from build123d import *

# Parameters (mm, degrees)
BOSS_EXTRUDE1_START = -242.545742
SKETCH1_R           = 25
BOSS_EXTRUDE1_DEPTH = 21.000001
BOSS_EXTRUDE2_START = -1.7
SKETCH4_R           = 25
SKETCH4_R_2         = 17
BOSS_EXTRUDE2_DEPTH = 1.7
FILLET1_R           = 4


with BuildPart() as part:
    # Sketch1 → Boss-Extrude1 (new body)
    with BuildSketch(Plane.XY.offset(BOSS_EXTRUDE1_START)):
        with Locations(Location((0, 0, 0), (0, 0, 270))):
            Circle(SKETCH1_R)
        with BuildLine():
            Line((-21.875959298, -8.922578372), (-20.951151281, -10.918757254))
            Line((-20.951151281, -10.918757254), (-20.019493054, -10.487130107))
            ThreePointArc((-20.019493054, -10.487130107), (-13.008740953, -18.480602231), (-3.118771073, -22.383772403))
            Line((-3.118771073, -22.383772403), (-3.210800112, -23.40642567))
            Line((-3.210800112, -23.40642567), (-1.019654481, -23.603607875))
            Line((-1.019654481, -23.603607875), (-0.927625442, -22.580954609))
            ThreePointArc((-0.927625442, -22.580954609), (9.500300533, -20.506201252), (17.825529997, -13.892821179))
            Line((17.825529997, -13.892821179), (18.665159186, -14.483847298))
            Line((18.665159186, -14.483847298), (19.931496801, -12.684850621))
            Line((19.931496801, -12.684850621), (19.091867612, -12.093824502))
            ThreePointArc((19.091867612, -12.093824502), (22.509041486, -2.025599021), (20.94430107, 8.490951224))
            Line((20.94430107, 8.490951224), (21.875959298, 8.922578372))
            Line((21.875959298, 8.922578372), (20.951151281, 10.918757254))
            Line((20.951151281, 10.918757254), (20.019493054, 10.487130107))
            ThreePointArc((20.019493054, 10.487130107), (13.008740953, 18.480602231), (3.118771073, 22.383772403))
            Line((3.118771073, 22.383772403), (3.210800112, 23.40642567))
            Line((3.210800112, 23.40642567), (1.019654481, 23.603607875))
            Line((1.019654481, 23.603607875), (0.927625442, 22.580954609))
            ThreePointArc((0.927625442, 22.580954609), (-9.500300533, 20.506201252), (-17.825529997, 13.892821179))
            Line((-17.825529997, 13.892821179), (-18.665159186, 14.483847298))
            Line((-18.665159186, 14.483847298), (-19.931496801, 12.684850621))
            Line((-19.931496801, 12.684850621), (-19.091867612, 12.093824502))
            ThreePointArc((-19.091867612, 12.093824502), (-22.509041486, 2.025599021), (-20.94430107, -8.490951224))
            Line((-20.94430107, -8.490951224), (-21.875959298, -8.922578372))
        make_face(mode=Mode.SUBTRACT)
    extrude(amount=BOSS_EXTRUDE1_DEPTH)

    # Sketch4 → Boss-Extrude2 (add)
    with BuildSketch(Plane.XY.offset(-221.545741472).offset(BOSS_EXTRUDE2_START)):
        with Locations(Location((0, 0, 0), (0, 0, 270))):
            Circle(SKETCH4_R)
        Circle(SKETCH4_R_2, mode=Mode.SUBTRACT)
    extrude(amount=BOSS_EXTRUDE2_DEPTH)

    # Fillet1
    fillet1_edges = [part.edges().sort_by_distance(p)[0] for p in [
        (0, 25, -221.545741),
    ]]
    fillet(fillet1_edges, radius=FILLET1_R)


solid = part.part
Could you check a few things on this model? Use its own coordinates, in mm. A direction names the side the tool comes from. Give positions to 0.01 mm unless a question says otherwise; leave off trailing zeros. Order: outer loops, then holes, each group sorted by start corner. A loop starts at its lowest first (then second) coordinate and runs counter-clockwise, first axis right, second up. Notation, with made-up numbers: (44, -11.5) -> (57, -11.5) arc R24 ccw to (57, 1.5) -> close; hole circle Ø6 at (85, -15.5). An arc over 180 degrees is marked (long way). Answer in a Markdown table with one row per item. Add a question column.
Item 1: I'm going to push flat-ended pins straight in: P1, Ø10, axis at y = -14, z = -235, coming from the +X side; P2, Ø20.5, axis at x = 0, y = 0, coming from the +Z side; P3, Ø5, axis at x = 16, z = -224.5, coming from the +Y side; P4, Ø12, axis at x = -8, z = -235.5, coming from the -Y side. Where does each tip first touch, or does it pass through?
Item 2: Imagine slicing it at A-A (z = -226.75). List the corners of the cut face in (x, y) for me, and give its area (3 significant figures).
Item 3: We'd pull the mould along X, two halves only. Please class faces 1 (the flat face through (-13, 19, -242.546)), 2 (the cylindrical face through (7.509, -23.846, -234.165)), 3 (the flat face through (-15, -9, -223.246)): pulls with the +X half, pulls with the -X half, needs draft (parallel to the pull), parting line crosses it, or undercut.
Item 4: For faces 4 (the flat face through (-17.3, 0.1, -221.546)), 5 (the cylindrical face through (-9.36, 20.57, -233.03)), which set-ups out of +Z, -Z, +X, -X, +Y, -Y let a thin tool reach every point of the face, with its end or its side?
Item 5: Please list where these lines run through material, in increasing order: probe 1 along Y at (x, z) = (0, -222.35); probe 2 along Z at (x, y) = (-17, 6); probe 3 along X at (y, z) = (-17, -231.25).
Result:
| question | item | result |
|---|---|---|
| 1 | P1 | x = 23.32 |
| 1 | P2 | through |
| 1 | P3 | y = 20.97 |
| 1 | P4 | y = -24.92 |
| 2 | outline | circle Ø50 at (0, 0); hole (-21.88, -8.92) -> (-20.95, -10.92) -> (-20.02, -10.49) arc R22.6 ccw to (-3.12, -22.38) -> (-3.21, -23.41) -> (-1.02, -23.6) -> (-0.93, -22.58) arc R22.6 ccw to (17.83, -13.89) -> (18.67, -14.48) -> (19.93, -12.68) -> (19.09, -12.09) arc R22.6 ccw to (20.94, 8.49) -> (21.88, 8.92) -> (20.95, 10.92) -> (20.02, 10.49) arc R22.6 ccw to (3.12, 22.38) -> (3.21, 23.41) -> (1.02, 23.6) -> (0.93, 22.58) arc R22.6 ccw to (-17.83, 13.89) -> (-18.67, 14.48) -> (-19.93, 12.68) -> (-19.09, 12.09) arc R22.6 ccw to (-20.94, -8.49) -> close |
| 2 | area | 346 mm2 |
| 3 | face 1 | needs draft |
| 3 | face 2 | parting line crosses it |
| 3 | face 3 | undercut |
| 4 | face 4 | +Z, +X, -X, +Y, -Y |
| 4 | face 5 | -Z |
| 5 | probe 1 | -23.41 to -17, 17 to 23.41 |
| 5 | probe 2 | -223.25 to -221.55 |
| 5 | probe 3 | -18.33 to -14.89, 14.89 to 18.33 |
